The figure shows three views and two pictorial views of one solid part (mm, origin at its lowest corner). Answer the questions. A direction names the side the tool comes from. Coordinates: 2 decimals unless noted, no trailing zeros. Loops run counter-clockwise (first coordinate to the right, second up) from the corner with the lowest first, then second, coordinate; pieces in that order, holes last. Notation, with made-up numbers: M -25.75,17.5 L 1.25,17.5 A29 ccw 1.25,38.5 Z; hole C 32,-2.5 d6. An arc over 180 degrees is marked long. One line per item, written item: value. Start each with the question number.
1. Flat-ended cylindrical pins translate along their axes: pin 1 (1.9 mm diameter, centred on x = 125, z = 9, fed in from +Y); pin 2 (3 mm diameter, centred on x = 57.5, y = 35, fed in from -Z); pin 3 (1.9 mm diameter, centred on x = 125, z = 13, fed in from -Y). Find the tip coordinate at first contact, or state that the pin passes through.
2. Determine the mould class of the marked faces 1, 2, 3 and 4 for opening direction Y: +Y half, -Y half, draft (parallel to the pull), parting line (faces both ways), or undercut.
3. The part is cut by section D-D (y = 115.5). Write down the section's boundary in (x, z), then the cut area to 3 significant figures.
4. Consider probe 1 along X at (y, z) = (8.5, 12.5); probe 2 along Y at (x, z) = (68, 31) (1 decimal); probe 3 along Z at (x, y) = (23, 20). Determine where each line is inside the solid, lowest interval first.
5. The part is cut by section B-B (y = 43). Write down the section's boundary in (x, z).
6. For the marked faces 5 and 6, determine the directions among +Z, -Z, +X, -X, +Y, -Y from which every point of the face is accessible in a straight line to the end or side of a thin tool.
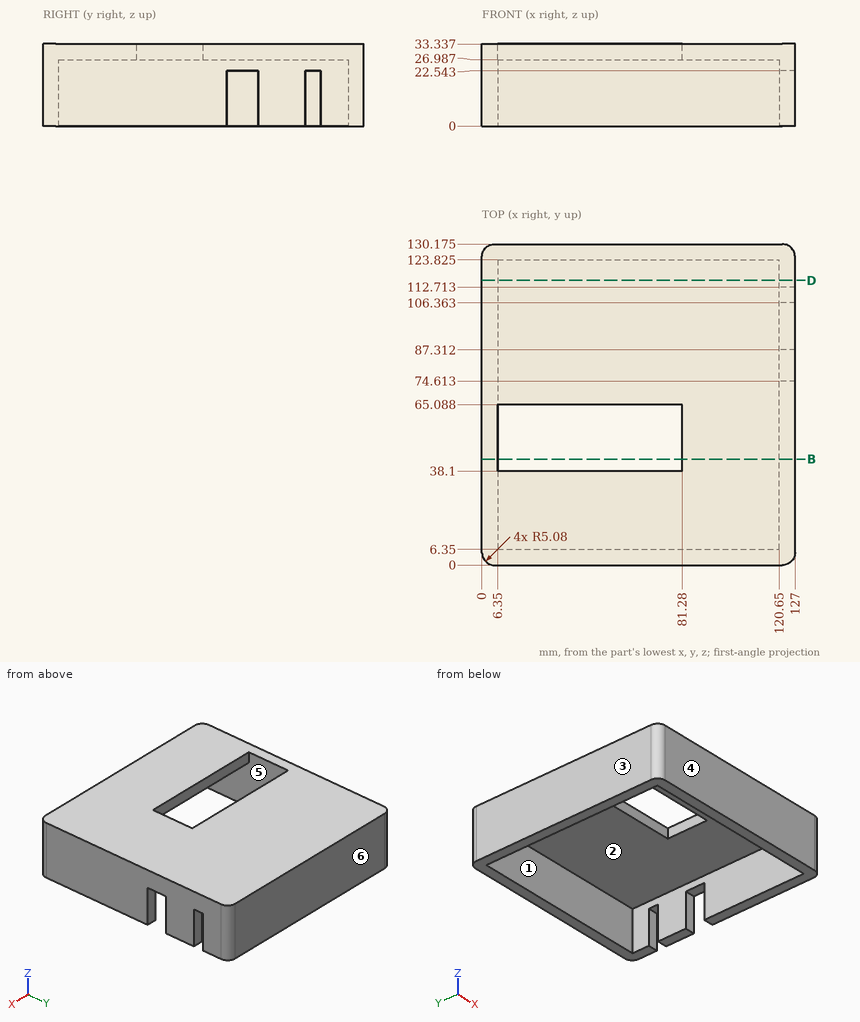
Answer block:
1. pin 1: stops at y = 129.71
1. pin 2: stops at z = 26.99
1. pin 3: stops at y = 0.47
2. face 1: undercut
2. face 2: undercut
2. face 3: draft
2. face 4: -Y half
3. outline: M 0,0 L 6.35,0 L 6.35,26.99 L 120.65,26.99 L 120.65,0 L 127,0 L 127,33.34 L 0,33.34 Z
3. area: 1,150 mm2
4. probe 1: x = 0 to 6.35, 120.65 to 127
4. probe 2: y = 0 to 38.1, 65.1 to 130.2
4. probe 3: z = 26.99 to 33.34
5. outline: M 0,0 L 6.35,0 L 6.35,33.34 L 0,33.34 Z; M 81.28,26.99 L 120.65,26.99 L 120.65,0 L 127,0 L 127,33.34 L 81.28,33.34 Z
6. face 5: -Z
6. face 6: +Z, -Z, +X, -X, +Y
